Geometry check sheet. Reference: drawing and pictorial views, mm from the part's lowest x, y, z. A direction names the side the tool comes from. Round coordinates to 2 decimals unless told otherwise and drop trailing zeros. Loops run counter-clockwise (first coordinate to the right, second up) from the corner with the lowest first, then second, coordinate; pieces in that order, holes last. Notation, with made-up numbers: M 78.25,73.5 L 82.25,73.5 A25 ccw 82.25,100.5 Z; hole C 19,83 d7. An arc over 180 degrees is marked long. One line per question, with ' | ' between items. Start each with the question number.
(1) Section check D-D (y = 14.5). Record the boundary of the cut face in (x, z), and give its area (3 significant figures).
(2) Go/stop test with flat-tipped pins: P1, Ø0.8, axis at x = 30, z = 1, coming from the -Y side; P2, Ø1.2, axis at y = 0.5, z = 1.5, coming from the -X side; P3, Ø1.5, axis at x = 16, z = 1.5, coming from the +Y side; P4, Ø1.6, axis at x = 1.5, y = 14.5, coming from the +Z side. Record where each tip stops, or that it passes through.
(3) Thickness scan on probe 1 along Y at (x, z) = (29.5, 1.55); probe 2 along X at (y, z) = (18, 0.2); probe 3 along Y at (x, z) = (4.5, 2.05). Record the ranges inside material, lowest first. Write a range as [from, to].
(4) Section check C-C (z = 1.7). Record the boundary of the cut face in (x, y).
(5) Draft check along Y on the marked faces 1, 2, 3 and 4. Enter one of: +Y half, -Y half, draft (parallel to the pull), parting line (faces both ways), or undercut.
(6) Tool access check on the marked faces 5, 6, 7, 8 and 9. Record the directions out of +Z, -Z, +X, -X, +Y, -Y that give a thin tool (end or side, any length) a straight path to the whole face; none if there is none.
(7) Section check A-A (y = 2). Record the boundary of the cut face in (x, z), and give its area (3 significant figures).
(8) Section check B-B (x = 13). Record the boundary of the cut face in (y, z).
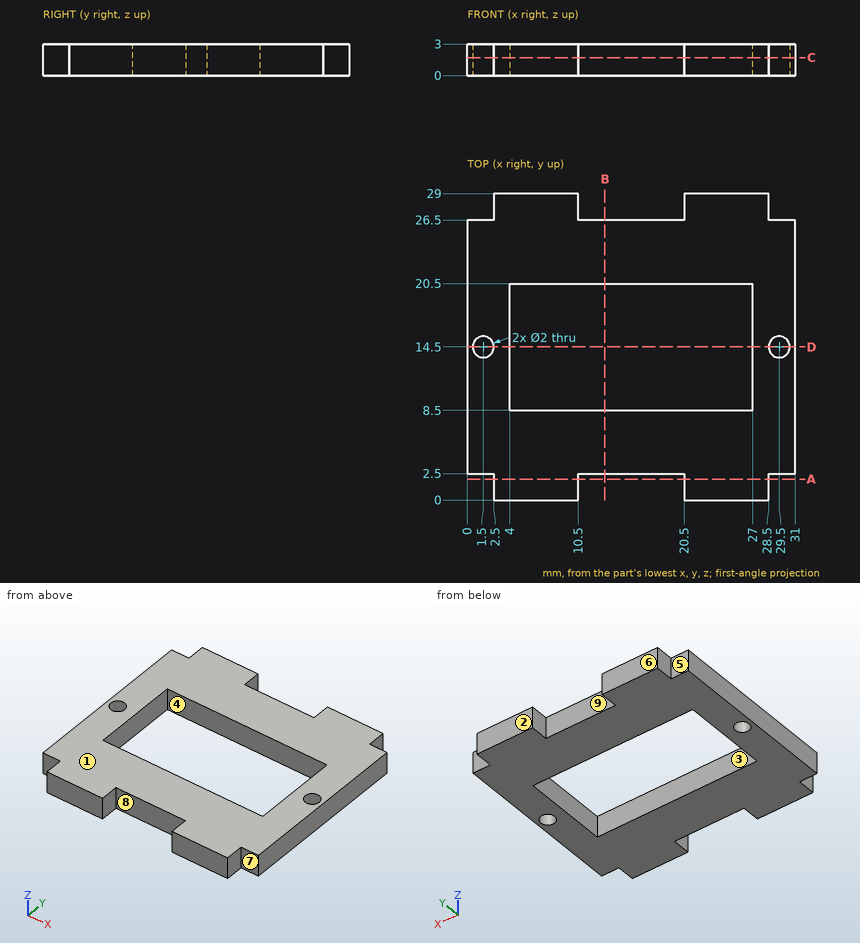
The answers:
1) outline: M 0,0 L 0.5,0 L 0.5,3 L 0,3 Z; M 2.5,0 L 4,0 L 4,3 L 2.5,3 Z; M 27,0 L 28.5,0 L 28.5,3 L 27,3 Z; M 30.5,0 L 31,0 L 31,3 L 30.5,3 Z | area: 12.0 mm²
2) P1: y = 2.5 | P2: x = 2.5 | P3: y = 26.5 | P4: through
3) probe 1: [2.5, 13.5], [15.5, 26.5] | probe 2: [0, 4], [27, 31] | probe 3: [0, 8.5], [20.5, 29]
4) outline: M 0,2.5 L 2.5,2.5 L 2.5,0 L 10.5,0 L 10.5,2.5 L 20.5,2.5 L 20.5,0 L 28.5,0 L 28.5,2.5 L 31,2.5 L 31,26.5 L 28.5,26.5 L 28.5,29 L 20.5,29 L 20.5,26.5 L 10.5,26.5 L 10.5,29 L 2.5,29 L 2.5,26.5 L 0,26.5 Z; hole C 1.5,14.5 d2; hole M 4,8.5 L 27,8.5 L 27,20.5 L 4,20.5 Z; hole C 29.5,14.5 d2
5) face 1: draft | face 2: +Y half | face 3: undercut | face 4: undercut
6) face 5: +Z, -Z, -X, +Y | face 6: +Z, -Z, +X, -X, +Y | face 7: +Z, -Z, +X, -Y | face 8: +Z, -Z, -Y | face 9: +Z, -Z, +Y
7) outline: M 2.5,0 L 10.5,0 L 10.5,3 L 2.5,3 Z; M 20.5,0 L 28.5,0 L 28.5,3 L 20.5,3 Z | area: 48.0 mm²
8) outline: M 2.5,0 L 8.5,0 L 8.5,3 L 2.5,3 Z; M 20.5,0 L 26.5,0 L 26.5,3 L 20.5,3 Z
